```python
from build123d import *

# Parameters (mm, degrees)
F0_W     = 25
F0_H     = 25
F0_W_2   = 19
F0_H_2   = 19
F1_DEPTH = 211
F2_R     = 1
F3_R     = 3
F5_DEPTH = 25.001
F7_D     = 6


with BuildPart() as f1:
    # F0 (on Top) → F1 (new body)
    with BuildSketch(Plane.XY):
        Rectangle(F0_W, F0_H)
        Rectangle(F0_W_2, F0_H_2, mode=Mode.SUBTRACT)
    extrude(amount=F1_DEPTH)

    # F2
    f2_edges = [f1.edges().sort_by_distance(p)[0] for p in [
        (-9.5, -9.5, 105.5),
        (-9.5, 9.5, 105.5),
        (9.5, 9.5, 105.5),
        (9.5, -9.5, 105.5),
    ]]
    fillet(f2_edges, radius=F2_R)

    # F3
    f3_edges = [f1.edges().sort_by_distance(p)[0] for p in [
        (-12.5, 12.5, 105.5),
        (-12.5, -12.5, 105.5),
        (12.5, 12.5, 105.5),
        (12.5, -12.5, 105.5),
    ]]
    fillet(f3_edges, radius=F3_R)

    # F4 (on face) → F5 (cut, through all)
    with BuildSketch(Plane.XZ.offset(12.5)):
        Polygon((-9.5, 211), (-9.5, 208), (9.5, 189), (9.5, 211), align=None)
        Polygon((-9.5, 211), (-12.5, 211), (-9.5, 208), align=None)
        Polygon((9.5, 211), (9.5, 189), (12.5, 186), (12.5, 211), align=None)
    extrude(amount=-F5_DEPTH, mode=Mode.SUBTRACT)

    # F7 (through all)
    with Locations(Plane(origin=(-12.5, 0, 0), x_dir=(0, -1, 0), z_dir=(-1, 0, 0))):
        with Locations((0, 12.5), (0, 52.5)):
            Hole(F7_D / 2)


solid = f1.part
```
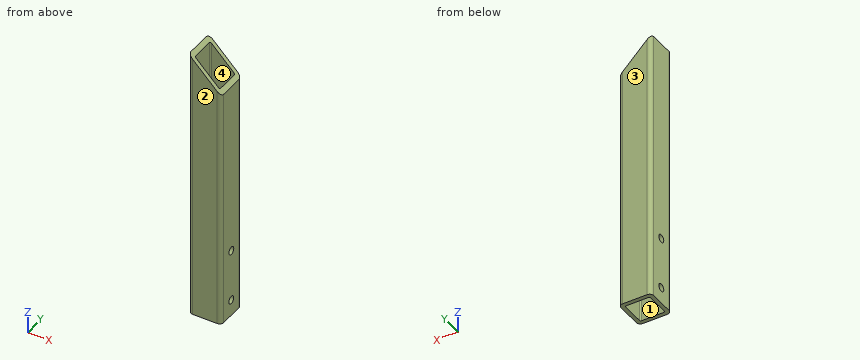
Here's how the part is built. I have some questions about the finished solid (model axes, mm). Face numbers are marked on the shaded views. A direction names the side the tool comes from. Coordinates: 2 decimals unless noted, no trailing zeros. Loops run counter-clockwise (first coordinate to the right, second up) from the corner with the lowest first, then second, coordinate; pieces in that order, holes last. Notation, with made-up numbers: (8.5, -16.75) - (22.5, -16.75) arc R24 ccw to (22.5, 12.25) - close; hole circle Ø1 at (-10.5, 0.25). An arc over 180 degrees is marked (long way). Return JSON: item names as keys, results as strings. Group by question number.
Item 1: Will this pin go through, and if not, where does the flat tip stop? P1, Ø5, axis at y = 0, z = 12.5, coming from the -X side.
Item 2: If we section it at C-C on x = -1.25: Write out the boundary of the cut face in (y, z), and give its area (3 significant figures).
Item 3: I need wall thicknesses on line 1 (Y direction, x = -0.5, z = 197); line 2 (Z direction, x = 10.1, y = 0). Which ranges of each line are inside material? Lowest first, please. Write a range as from..to.
Item 4: If we section it at B-B on y = 0: Write out the boundary of the cut face in (x, z), and give its area (3 significant figures).
Item 5: We'd pull the mould along X, two halves only. Please class the marked faces 1 and 2: +X half, -X half, draft (parallel to the pull), parting line (faces both ways), or undercut.
Item 6: If we section it at A-A on z = 134.5: Write out the boundary of the cut face in (x, y).
Item 7: On a 3-axis mill with a long thin cutter (end or side, diameter ignored), from which of +Z, -Z, +X, -X, +Y, -Y can I reach the whole of each face in a straight line? I mean the marked faces 3 and 4. Say none if no direction works.
Item 8: If we section it at D-D on z = 12.5: Write out the boundary of the cut face in (x, y), and give its area (3 significant figures).
Calculated:
{
 "1": {"P1": "passes through"},
 "2": {"outline": "(-12.5, 0) - (-9.5, 0) - (-9.5, 199.75) - (-12.5, 199.75) - close; (9.5, 0) - (12.5, 0) - (12.5, 199.75) - (9.5, 199.75) - close", "area": "1,200 mm^2"},
 "3": {"line 1": "y = -12.5..-9.5, 9.5..12.5", "line 2": "z = 0..9.5, 15.5..49.5, 55.5..188.4"},
 "4": {"outline": "(-12.5, 0) - (-9.5, 0) - (-9.5, 9.5) - (-12.5, 9.5) - close; (-12.5, 15.5) - (-9.5, 15.5) - (-9.5, 49.5) - (-12.5, 49.5) - close; (-12.5, 55.5) - (-9.5, 55.5) - (-9.5, 208) - (-12.5, 211) - close; (9.5, 0) - (12.5, 0) - (12.5, 9.5) - (9.5, 9.5) - close; (9.5, 15.5) - (12.5, 15.5) - (12.5, 49.5) - (9.5, 49.5) - close; (9.5, 55.5) - (12.5, 55.5) - (12.5, 186) - (9.5, 189) - close", "area": "1,120 mm^2"},
 "5": {"face 1": "undercut", "face 2": "draft"},
 "6": {"outline": "(-12.5, -9.5) arc R3 ccw to (-9.5, -12.5) - (9.5, -12.5) arc R3 ccw to (12.5, -9.5) - (12.5, 9.5) arc R3 ccw to (9.5, 12.5) - (-9.5, 12.5) arc R3 ccw to (-12.5, 9.5) - close; hole (-9.5, -8.5) arc R1 ccw to (-8.5, -9.5) - (8.5, -9.5) arc R1 ccw to (9.5, -8.5) - (9.5, 8.5) arc R1 ccw to (8.5, 9.5) - (-8.5, 9.5) arc R1 ccw to (-9.5, 8.5) - close"},
 "7": {"face 3": "+Z, -Z, +X, -X, +Y", "face 4": "+Z, -Z"},
 "8": {"outline": "(-12.5, -9.5) arc R3 ccw to (-9.5, -12.5) - (9.5, -12.5) arc R3 ccw to (12.5, -9.5) - (12.5, -3) - (9.5, -3) - (9.5, -8.5) arc R1 cw to (8.5, -9.5) - (-8.5, -9.5) arc R1 cw to (-9.5, -8.5) - (-9.5, -3) - (-12.5, -3) - close; (-12.5, 3) - (-9.5, 3) - (-9.5, 8.5) arc R1 cw to (-8.5, 9.5) - (8.5, 9.5) arc R1 cw to (9.5, 8.5) - (9.5, 3) - (12.5, 3) - (12.5, 9.5) arc R3 ccw to (9.5, 12.5) - (-9.5, 12.5) arc R3 ccw to (-12.5, 9.5) - close", "area": "221 mm^2"}
}
